Geometry: final body of the model. Coordinates: model frame, mm. Face numbers are marked on the shaded views. Give positions to 0.01 mm unless a question says otherwise; leave off trailing zeros. Write each loop counter-clockwise with the first axis right and the second up, starting at its lowest first coordinate (ties: lowest second). Pieces come first, ordered by that corner, then holes. Notation, with made-up numbers: (28, 53) - (45, 53) arc R6 ccw to (45, 59) - close; hole circle Ø9 at (-36, 10). An arc over 180 degrees is marked (long way). Return JSON: item names as keys, results as strings.
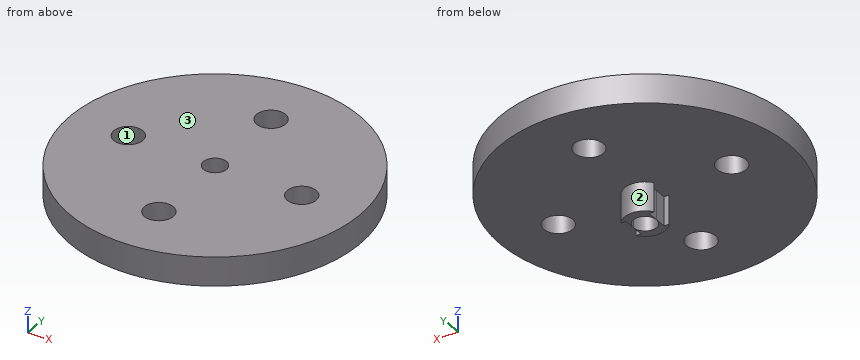
Autodesk Inventor part; units mm, degrees
ref_plane "YZ Plane" through (0, 0, 0) normal (1, 0, 0) x (0, 1, 0)
ref_plane "XZ Plane" through (0, 0, 0) normal (0, 1, 0) x (-1, 0, 0)
ref_plane "XY Plane" through (0, 0, 0) normal (0, 0, 1) x (1, 0, 0)
sketch "Sketch1" plane through (0, 0, 0) normal (0, 0, 1) x (1, 0, 0)
  circle A0 centre (0, 0) radius 2
  circle A1 centre (0, 0) radius 25
  circle A2 centre (0, 0) radius 3.5
  line L0 (-2, -2.8723) -> (-2, 2.8723)
  line L1 (-2.8723, 2) -> (2.8723, 2)
  line L2 (-2.8723, -2) -> (2.8723, -2)
  line L3 (2, -2.8723) -> (2, 2.8723)
  point P0 (2, -2)
  point P1 (2, 0)
  point P2 (-2, 0)
  point P3 (-2, -2)
  point P4 (2, 2)
  point P5 (-2, 2)
  dimension "d4" = 7
  dimension "d0" = 4
  dimension "d1" = 50
extrude "Extrusion1" add sketch "Sketch1" along normal blind 5 contours L3 L2 A0 | L3 L1 A2 L2 | A0 L1 L3 | A0 L0 L1 | L1 L0 A2 L3 | L2 L0 A0 | L2 L3 A2 L0 | L2 A2 L3 | L3 A2 L1 | L0 L2 A2 L1 | L1 A2 L0 | L0 A2 L2 | A1
extrude "Extrusion2" add sketch "Sketch1" against normal blind 5 contours L3 L2 A0 | A0 L1 L3 | A0 L0 L1 | L1 L0 A2 L3 | L2 L0 A0 | L2 L3 A2 L0 | L2 A2 L3 | L3 A2 L1 | L1 A2 L0 | L0 A2 L2
sketch "Sketch2" plane through (0, 0, 5) normal (0, 0, 1) x (1, 0, 0)
  circle A0 centre (0, 0) radius 2
  circle A1 centre (0, 0) radius 15
  circle A2 centre (-15, 0) radius 2.5
  circle A3 centre (0, 15) radius 2.5
  circle A4 centre (15, 0) radius 2.5
  circle A5 centre (0, -15) radius 2.5
  dimension "d7" = 30
  dimension "d8" = 5
  dimension "d9" = 5
  dimension "d10" = 5
  dimension "d11" = 5
extrude "Extrusion3" cut sketch "Sketch2" against normal through all contours A1 A4 | A1 A4 | A3 A1 | A1 A3 | A5 A1 | A1 A5 | A2 A1 | A1 A2
Q1. Section query A-A, the plane x = -15. Return the cut outline in (y, z).
Answer key:
{"outline": "(-20, 0) - (-2.5, 0) - (-2.5, 5) - (-20, 5) - close; (2.5, 0) - (20, 0) - (20, 5) - (2.5, 5) - close"}
Q2. Section query C-C, the plane z = 2.5. Return the cut outline in (x, y).
Answer key:
{"outline": "circle Ø50 at (0, 0); hole circle Ø5 at (-15, 0); hole circle Ø5 at (0, -15); hole circle Ø5 at (0, 15); hole circle Ø4 at (0, 0); hole circle Ø5 at (15, 0)"}
Q3. Material intervals for probe 1 along Y at (x, z) = (0.5, 4.25) (1 decimal); probe 2 along Z at (x, y) = (-21, 6.5); probe 3 along Y at (x, z) = (15, 2.15), sorted ascending. Write a range as [from, to].
Answer key:
{"probe 1": "y = [-25, -17.4], [-12.6, -1.9], [1.9, 12.6], [17.4, 25]", "probe 2": "z = [0, 5]", "probe 3": "y = [-20, -2.5], [2.5, 20]"}
Q4. Mould query, pull axis X, two halves, no side actions, for the marked faces 1, 2 and 3. Classes: pulls with the +X half, pulls with the -X half, needs draft (parallel to the pull), parting line crosses it, or undercut.
Answer key:
{"face 1": "undercut", "face 2": "parting line crosses it", "face 3": "needs draft"}
Q5. Section query D-D, the plane x = 0. Return the cut outline in (y, z).
Answer key:
{"outline": "(-25, 0) - (-17.5, 0) - (-17.5, 5) - (-25, 5) - close; (-12.5, 0) - (-3.5, 0) - (-3.5, -5) - (-2, -5) - (-2, 5) - (-12.5, 5) - close; (2, -5) - (3.5, -5) - (3.5, 0) - (12.5, 0) - (12.5, 5) - (2, 5) - close; (17.5, 0) - (25, 0) - (25, 5) - (17.5, 5) - close"}
Q6. Pin query (flat end, axial travel): P1, Ø0.7, axis at x = -2.5, z = -3.5, coming from the +Y side; P2, Ø6, axis at x = 3.5, z = -1, coming from the +Y side; P3, Ø5, axis at y = 8, z = 4, coming from the -X side; P4, Ø15, axis at x = 10, y = -3.5, coming from the -Z side. Return the tip coordinate at first contact, or that it passes through.
Answer key:
{"P1": "stops at y = 2.76", "P2": "stops at y = 24.99", "P3": "stops at x = -24.39", "P4": "stops at z = -5"}
